Design review of the part shown in the three views and the two pictorial views. Dimensions are in mm from the part's minimum x, y and z. Coordinates: 2 decimals unless noted, no trailing zeros. Order: outer loops, then holes, each group sorted by start corner. A loop starts at its lowest first (then second) coordinate and runs counter-clockwise, first axis right, second up. Notation, with made-up numbers: (64.25, -15.75) -> (74.25, -15.75) arc R24 cw to (74.25, 15.25) -> close; hole circle Ø5 at (13, -37). An arc over 180 degrees is marked (long way). Write item = value, one per line. Start each with the question number.
1) Wall thickness on probe 1 along X at (y, z) = (6.35, 1.15); probe 2 along Y at (x, z) = (6.35, 1.7): over which ranges is each line inside the solid? List them lowest first. Write a range as [from, to].
2) Consider section C-C on z = 2.4. Give the boundary of the cut face in (x, y), and give its area (3 significant figures).
3) Draft analysis for pull direction X (two halves, no side actions). For the marked faces 1, 2, 3 and 4, state which applies: +X half, -X half, draft (parallel to the pull), parting line (faces both ways), or undercut.
4) Consider section A-A on y = 6.35. Give the boundary of the cut face in (x, z) (1 decimal), and give its area (3 significant figures).
5) Consider section B-B on x = 6.35. Give the boundary of the cut face in (y, z) (1 decimal), and give its area (3 significant figures).
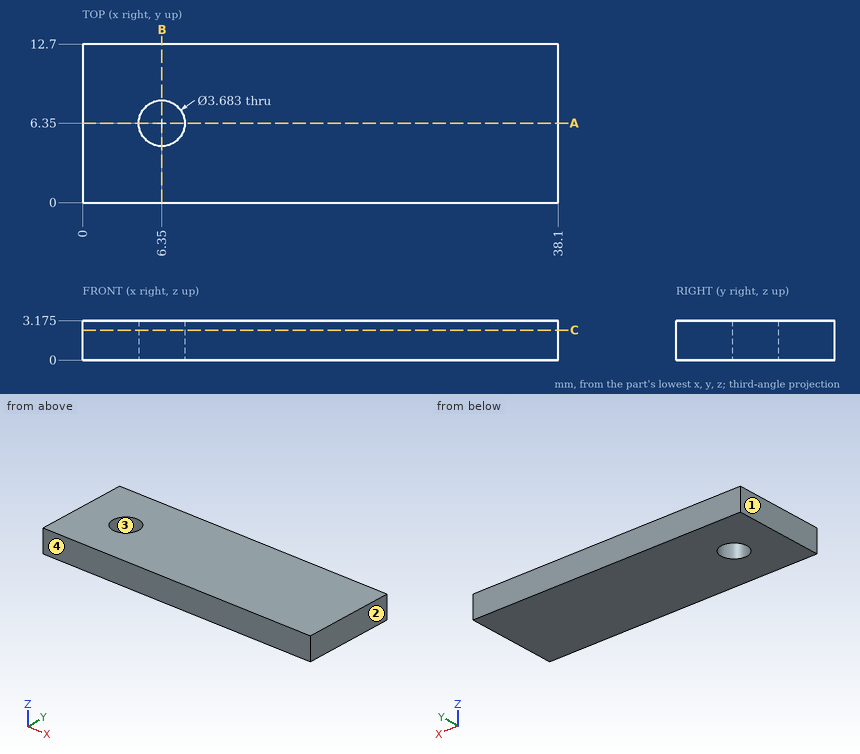
Answer sheet:
q1.probe_1 = [0, 4.51], [8.19, 38.1]
q1.probe_2 = [0, 4.51], [8.19, 12.7]
q2.outline = (0, 0) -> (38.1, 0) -> (38.1, 12.7) -> (0, 12.7) -> close; hole circle Ø3.68 at (6.35, 6.35)
q2.area = 473 mm2
q3.face_1 = -X half
q3.face_2 = +X half
q3.face_3 = undercut
q3.face_4 = draft
q4.outline = (0, 0) -> (4.5, 0) -> (4.5, 3.2) -> (0, 3.2) -> close; (8.2, 0) -> (38.1, 0) -> (38.1, 3.2) -> (8.2, 3.2) -> close
q4.area = 109 mm2
q5.outline = (0, 0) -> (4.5, 0) -> (4.5, 3.2) -> (0, 3.2) -> close; (8.2, 0) -> (12.7, 0) -> (12.7, 3.2) -> (8.2, 3.2) -> close
q5.area = 28.6 mm2
